Part model, mm, in its own coordinate system. Face numbers are marked on the shaded views. A direction names the side the tool comes from. Coordinates: 2 decimals unless noted, no trailing zeros. Loops run counter-clockwise (first coordinate to the right, second up) from the corner with the lowest first, then second, coordinate; pieces in that order, holes last. Notation, with made-up numbers: (-31.75, 72) -> (-9.75, 72) arc R17 cw to (-9.75, 101) -> close; hole circle Ø2 at (82.25, 59.5). An arc over 180 degrees is marked (long way). One line per item, written item: value. Start each with the question number.
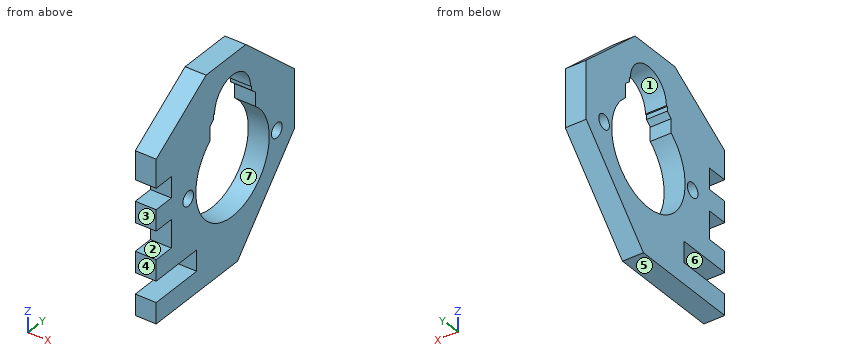
from build123d import *

# Parameters (mm, degrees)
SKETCH1_R           = 2.1
BOSS_EXTRUDE1_DEPTH = 6


with BuildPart() as part:
    # Sketch1 → Boss-Extrude1 (new body)
    with BuildSketch(Plane(origin=(0, 0, 0), x_dir=(0, 0, -1), z_dir=(1, 0, 0))):
        Polygon((10.014395287, -23.10816726), (1.8561273, -23.10816726), (-10.880328259, -3.400467914), (-10.880328259, 12.294369708), (6.488451552, 31.621864486), (23.016962848, 31.621864486), (48.014395287, 9.017628036), (48.014395287, -23.10816726), (42.014395287, -23.10816726), (42.014395287, -7.10816726), (36.014395287, -7.10816726), (36.014395287, -23.10816726), (30.014395287, -23.10816726), (30.014395287, -17.128409951), (22.014395287, -17.128409951), (22.014395287, -23.10816726), (16.014395287, -23.10816726), (16.014395287, -17.10816726), (10.014395287, -17.10816726), align=None)
        with Locations((19.8561273, -10.445316887)):
            Circle(SKETCH1_R, mode=Mode.SUBTRACT)
        with Locations((19.8561273, 24.554683113)):
            Circle(SKETCH1_R, mode=Mode.SUBTRACT)
        with BuildLine():
            Line((4.487310299, -1.945316887), (3.1561273, -0.445316887))
            Line((3.1561273, -0.445316887), (1.8561273, -0.445316887))
            Line((1.8561273, -0.445316887), (1.8561273, -0.041769088))
            ThreePointArc((1.8561273, -0.041769088), (-5.240324902, 7.054683113), (1.8561273, 14.151135315))
            Line((1.8561273, 14.151135315), (1.8561273, 14.554683113))
            Line((1.8561273, 14.554683113), (3.1561273, 14.554683113))
            Line((3.1561273, 14.554683113), (4.487310299, 16.054683113))
            Line((4.487310299, 16.054683113), (8.487310299, 16.054683113))
            ThreePointArc((8.487310299, 16.054683113), (34.3561273, 7.054683113), (8.487310299, -1.945316887))
            Line((8.487310299, -1.945316887), (4.487310299, -1.945316887))
        make_face(mode=Mode.SUBTRACT)
    extrude(amount=BOSS_EXTRUDE1_DEPTH)


solid = part.part
1) Slice it at D-D (x = 4.5). State how many separate pieces and enclosed holes the cut face has, then the cut area to 3 significant figures.
2) Pin check, flat tips, straight feed: pin 1 Ø3 at (x, y) = (2, -21) entering from +Z; pin 2 Ø1.8 at (x, y) = (3.5, -13.5) entering from +Z; pin 3 Ø3 at (x, z) = (2.5, -27) entering from -Y; pin 4 Ø8 at (y, z) = (3.5, -29) entering from +X. Stop position of each tip, or through.
3) Slice it at C-C (y = -19). Give the cut face in (x, z).
4) Slice it at B-B (y = 20.5). Give the cut face in (x, z), then the cut area to 3 significant figures.
5) Slice it at A-A (z = -12.5). Give the cut face in (x, y).
6) Tool access for the marked faces 1, 2 and 3: list every direction of +Z, -Z, +X, -X, +Y, -Y with a clear straight run to the whole face (end or side of a thin tool).
7) Pull direction Z, two halves, no side cores. Call the marked faces 4, 5, 6 and 7: +Z half, -Z half, draft (parallel to the pull), parting line (faces both ways), or undercut.
8) Probe line 1 (Y direction, x = 1.4, z = -21); line 2 (Y direction, x = 5.3, z = -18); line 3 (Y direction, x = 3, z = -3). List the from-to ranges inside material, lowest first. Write a range as from..to.
Check sheet entries:
1. separate pieces: 1
1. enclosed holes: 3
1. area: 1,630 mm^2
2. pin 1: stops at z = 0.48
2. pin 2: stops at z = 4.93
2. pin 3: stops at y = -17.13
2. pin 4: passes through
3. outline: (0, -48.01) -> (6, -48.01) -> (6, -42.01) -> (0, -42.01) -> close; (0, -36.01) -> (6, -36.01) -> (6, -30.01) -> (0, -30.01) -> close; (0, -22.01) -> (6, -22.01) -> (6, -16.01) -> (0, -16.01) -> close; (0, -10.01) -> (6, -10.01) -> (6, 0.8) -> (0, 0.8) -> close
4. outline: (0, -35.32) -> (6, -35.32) -> (6, -25.29) -> (0, -25.29) -> close; (0, -14.43) -> (6, -14.43) -> (6, 3.51) -> (0, 3.51) -> close
4. area: 168 mm^2
5. outline: (0, -17.11) -> (6, -17.11) -> (6, -5.44) -> (0, -5.44) -> close; (0, 19.55) -> (6, 19.55) -> (6, 31.62) -> (0, 31.62) -> close
6. face 1: +X, -X
6. face 2: +X, -X, -Y
6. face 3: +Z, -Z, +X, -X, -Y
7. face 4: draft
7. face 5: -Z half
7. face 6: undercut
7. face 7: undercut
8. line 1: y = -23.11..-12.21, -8.68..-7.4, 21.51..22.79, 26.32..31.62
8. line 2: y = -23.11..-11.43, -9.46..-7.33, 21.44..23.57, 25.54..31.62
8. line 3: y = -23.11..-0.45, 14.55..27.74
